Build history of the part. All positions in model axes, mm. A direction names the side the tool comes from. Coordinates: 2 decimals unless noted, no trailing zeros. Write each loop counter-clockwise with the first axis right and the second up, starting at its lowest first coordinate (ties: lowest second). Pieces come first, ordered by that corner, then holes. Notation, with made-up numbers: (61.25, 15) -> (78.25, 15) arc R9 ccw to (78.25, 29) -> close; hole circle Ø1 at (-15.75, 74.5). An arc over 180 degrees is marked (long way). Write each question's results on one line, items separated by ' | '. Start each with the question number.
Q1. Saw through at B-B on x = 9.5. Give the cut face in (y, z), and give its area (3 significant figures).
Q2. Tool access for faces 1 (the face through (110, 33, 4)), 2 (the face through (99, 25, 2)): list every direction of +Z, -Z, +X, -X, +Y, -Y with a clear straight run to the whole face (end or side of a thin tool).
Q3. Saw through at D-D on y = 8.5. Give the cut face in (x, z), and give its area (3 significant figures).
Q4. Drill centre lines: line 1 (X direction, y = 13, z = 6.25); line 2 (Y direction, x = 17.5, z = 5); line 3 (Y direction, x = 43.5, z = 5.75). Where is each one in solid material? Low to high.
Q5. Two-plate mould, pull along Y, no slides. Class faces 3 (the face through (55, 18, 0)), 4 (the face through (62, 35, 4)), 5 (the face through (109, 1, 4)), 6 (the face through (80, 26, 1)): released by +Y, released by -Y, zero draft, split by the parting line, or undercut.
Q6. Saw through at A-A on y = 29. Give the cut face in (x, z).
Q7. Saw through at C-C on x = 61. Give the cut face in (y, z).
from build123d import *

# Parameters (mm, degrees)
F0_R     = 12.5
F1_DEPTH = 8


with BuildPart() as f1:
    # F0 (on Top) → F1 (new body)
    with BuildSketch(Plane.XY):
        with BuildLine():
            ThreePointArc((0, 17.5), (5.125631, 5.125631), (17.5, 0))
            Line((17.5, 0), (106, 0))
            ThreePointArc((106, 0), (109.535534, 1.464466), (111, 5))
            Line((111, 5), (111, 30))
            ThreePointArc((111, 30), (109.535534, 33.535534), (106, 35))
            Line((106, 35), (17.5, 35))
            ThreePointArc((17.5, 35), (5.125631, 29.874369), (0, 17.5))
        make_face()
        with Locations((17.5, 17.5)):
            Circle(F0_R, mode=Mode.SUBTRACT)
    extrude(amount=F1_DEPTH)

    # F2 (on face) → F3 (revolve, cut)
    with BuildSketch(Plane.XY.offset(8)):
        Polygon((105, 27), (99, 27), (99, 22.5), (99, 20.3), (99, 10.3), (102.5, 10.3), (102.5, 20.3), (106, 20.3), (106, 22.5), (105, 22.5), align=None)
    revolve(axis=Axis((99, 15.3, 8), (0, -1, 0)), mode=Mode.SUBTRACT)

    # F2 (on face) → F4 (revolve, cut)
    with BuildSketch(Plane.XY.offset(8)):
        Polygon((87, 27), (80, 27), (80, 25), (80, 20), (80, 7), (83.5, 7), (83.5, 20), (83.63197, 20), (87, 25), align=None)
    revolve(axis=Axis((80, 13.5, 8), (0, -1, 0)), mode=Mode.SUBTRACT)

    # F2 (on face) → F5 (revolve, cut)
    with BuildSketch(Plane.XY.offset(8)):
        Polygon((68, 27), (61, 27), (61, 25), (61, 20), (61, 7), (64.5, 7), (64.5, 20), (68, 25), align=None)
    revolve(axis=Axis((61, 13.5, 8), (0, -1, 0)), mode=Mode.SUBTRACT)

    # F2 (on face) → F6 (revolve, cut)
    with BuildSketch(Plane.XY.offset(8)):
        Polygon((49, 27), (42, 27), (42, 25), (42, 20), (42, 7), (45.5, 7), (45.5, 20), (49, 25), align=None)
    revolve(axis=Axis((42, 13.5, 8), (0, -1, 0)), mode=Mode.SUBTRACT)


solid = f1.part
Returned:
1) outline: (1.94, 0) -> (7.9, 0) -> (7.9, 8) -> (1.94, 8) -> close; (27.1, 0) -> (33.06, 0) -> (33.06, 8) -> (27.1, 8) -> close | area: 95.4 mm2
2) face 1: +Z, -Z, +X, +Y | face 2: +Z
3) outline: (2.49, 0) -> (8.83, 0) -> (8.83, 8) -> (2.49, 8) -> close; (26.17, 0) -> (111, 0) -> (111, 8) -> (83.5, 8) arc R3.5 cw to (76.5, 8) -> (64.5, 8) arc R3.5 cw to (57.5, 8) -> (45.5, 8) arc R3.5 cw to (38.5, 8) -> (26.17, 8) -> close | area: 672 mm2
4) line 1: x = 0.59 to 5.84, 29.16 to 38.97, 45.03 to 57.97, 64.03 to 76.97, 83.03 to 95.97, 102.03 to 111 | line 2: y = 0 to 5, 30 to 35 | line 3: y = 0 to 7, 27 to 35
5) face 3: zero draft | face 4: released by +Y | face 5: released by -Y | face 6: undercut
6) outline: (4.31, 0) -> (12.6, 0) -> (12.6, 8) -> (4.31, 8) -> close; (22.4, 0) -> (111, 0) -> (111, 8) -> (22.4, 8) -> close
7) outline: (0, 0) -> (35, 0) -> (35, 8) -> (27, 8) -> (27, 1) -> (25, 1) -> (20, 4.5) -> (7, 4.5) -> (7, 8) -> (0, 8) -> close
